from build123d import *

# Parameters (mm, degrees)
F0_W     = 76.2
F0_H     = 120.65
F0_R     = 2.5527
F1_DEPTH = 6.35
F2_R     = 9.525
F3_DEPTH = 6.35
F2_W     = 55.88
F2_H     = 43.18
F4_DEPTH = 5
F5_R     = 5.08
F6_W     = 69.85
F6_H     = 69.85
F6_W_2   = 62.23
F6_H_2   = 59.69
F7_DEPTH = 1.08458
F9_DEPTH = 5


# Not quite as in the source:
# - a length typed as a fraction of an inch, garbled in the dataset ("3 / 203.2 mm" for 3/8 in), is restored


with BuildPart() as f1:
    # F0 (on Top) → F1 (new body)
    with BuildSketch(Plane.XY):
        Rectangle(F0_W, F0_H)
        with Locations((-29.8323, -52.0573)):
            Circle(F0_R, mode=Mode.SUBTRACT)
        with Locations((29.8323, -52.0573)):
            Circle(F0_R, mode=Mode.SUBTRACT)
        with Locations((-29.8323, 52.0573)):
            Circle(F0_R, mode=Mode.SUBTRACT)
        with Locations((29.8323, 52.0573)):
            Circle(F0_R, mode=Mode.SUBTRACT)
    extrude(amount=F1_DEPTH)

    # F2 (on face) → F3 (cut)
    with BuildSketch(Plane.XY.offset(6.35)):
        Circle(F2_R)
    extrude(amount=-F3_DEPTH, mode=Mode.SUBTRACT)

    # F2 (on face) → F4 (cut)
    with BuildSketch(Plane.XY.offset(6.35)):
        with Locations((0, -1.27)):
            Rectangle(F2_W, F2_H)
        Circle(F2_R, mode=Mode.SUBTRACT)
    extrude(amount=-F4_DEPTH, mode=Mode.SUBTRACT)

    # F5
    f5_edges = [f1.edges().sort_by_distance(p)[0] for p in [
        (38.1, -60.325, 3.175),
        (38.1, 60.325, 3.175),
        (-38.1, 60.325, 3.175),
        (-38.1, -60.325, 3.175),
    ]]
    fillet(f5_edges, radius=F5_R)

    # F6 (on face) → F7 (cut)
    with BuildSketch(Plane.XY.offset(6.35)):
        Rectangle(F6_W, F6_H)
        Rectangle(F6_W_2, F6_H_2, mode=Mode.SUBTRACT)
    extrude(amount=-F7_DEPTH, mode=Mode.SUBTRACT)

    # F8 (on face) → F9 (cut)
    with BuildSketch(Plane.XY.offset(6.35)):
        Polygon((-25.7090758532, 20.32), (-20.905200392, 20.32), (-20.905200392, 22.5038137287), (27.94, 22.5038137287), (27.94, 26.3926647604), (-25.7090758532, 26.3926647604), align=None)
    extrude(amount=-F9_DEPTH, mode=Mode.SUBTRACT)


solid = f1.part
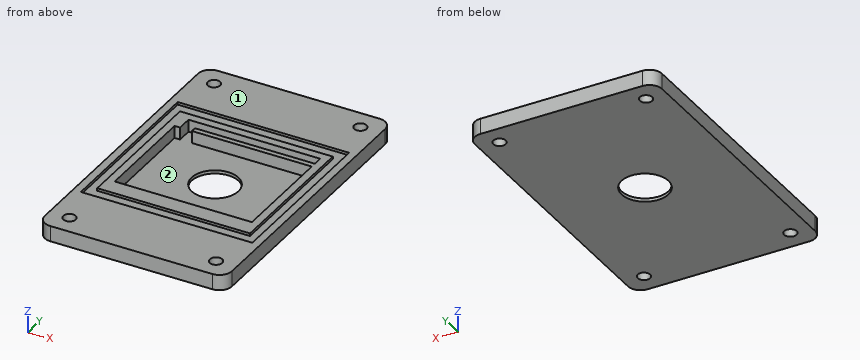
Design review of the part built by this model. Coordinates are the model's own, in mm. Face numbers are marked on the shaded views. Round coordinates to 2 decimals unless told otherwise and drop trailing zeros. Order: outer loops, then holes, each group sorted by start corner. A loop starts at its lowest first (then second) coordinate and runs counter-clockwise, first axis right, second up.
1) Consider section C-C (x = -11.5). State the section outline as (y, z) points (3 decimals).
The answers:
outline: (-60.325, 0) - (60.325, 0) - (60.325, 6.35) - (34.925, 6.35) - (34.925, 5.265) - (29.845, 5.265) - (29.845, 6.35) - (26.393, 6.35) - (26.393, 1.35) - (22.504, 1.35) - (22.504, 6.35) - (20.32, 6.35) - (20.32, 1.35) - (-22.86, 1.35) - (-22.86, 6.35) - (-29.845, 6.35) - (-29.845, 5.265) - (-34.925, 5.265) - (-34.925, 6.35) - (-60.325, 6.35) - close
2) Consider section A-A (y = 0). State the section outline as (x, z) points (3 decimals).
The answers:
outline: (-38.1, 0) - (-9.525, 0) - (-9.525, 1.35) - (-27.94, 1.35) - (-27.94, 6.35) - (-31.115, 6.35) - (-31.115, 5.265) - (-34.925, 5.265) - (-34.925, 6.35) - (-38.1, 6.35) - close; (9.525, 0) - (38.1, 0) - (38.1, 6.35) - (34.925, 6.35) - (34.925, 5.265) - (31.115, 5.265) - (31.115, 6.35) - (27.94, 6.35) - (27.94, 1.35) - (9.525, 1.35) - close
3) Consider section B-B (x = 0). State the section outline as (y, z) points (3 decimals).
The answers:
outline: (-60.325, 0) - (-9.525, 0) - (-9.525, 1.35) - (-22.86, 1.35) - (-22.86, 6.35) - (-29.845, 6.35) - (-29.845, 5.265) - (-34.925, 5.265) - (-34.925, 6.35) - (-60.325, 6.35) - close; (9.525, 0) - (60.325, 0) - (60.325, 6.35) - (34.925, 6.35) - (34.925, 5.265) - (29.845, 5.265) - (29.845, 6.35) - (26.393, 6.35) - (26.393, 1.35) - (22.504, 1.35) - (22.504, 6.35) - (20.32, 6.35) - (20.32, 1.35) - (9.525, 1.35) - close
4) For L1, parallel to Y at x = 0.5, z = 4.25 (3 decimals); L2, parallel to Y at x = -27, z = 4 (3 decimals); L3, parallel to X at y = 22, z = 1.5, list the stretches that pass through material, from the lowest coordinate up.
The answers:
L1: y = -60.325 to -22.86, 20.32 to 22.504, 26.393 to 60.325
L2: y = -60.325 to -22.86, 20.32 to 60.325
L3: x = -38.1 to -25.71, -20.91 to 38.1
5) Consider section D-D (z = 4.25). State the section outline as (x, y) points (3 decimals), plus the area to 3 significant figures.
The answers:
outline: (-38.1, -55.245) arc R5.08 ccw to (-33.02, -60.325) - (33.02, -60.325) arc R5.08 ccw to (38.1, -55.245) - (38.1, 55.245) arc R5.08 ccw to (33.02, 60.325) - (-33.02, 60.325) arc R5.08 ccw to (-38.1, 55.245) - close; hole circle Ø5.105 at (-29.832, -52.057); hole circle Ø5.105 at (-29.832, 52.057); hole (-27.94, -22.86) - (27.94, -22.86) - (27.94, 20.32) - (-20.905, 20.32) - (-20.905, 22.504) - (27.94, 22.504) - (27.94, 26.393) - (-25.709, 26.393) - (-25.709, 20.32) - (-27.94, 20.32) - close; hole circle Ø5.105 at (29.832, -52.057); hole circle Ø5.105 at (29.832, 52.057)
area: 6,460 mm2
6) Clearance check with a flat-ended pin moving along its axis: pin 1 Ø1.5 at (x, y) = (-6.5, 6.5) entering from +Z. State where the tip first meets the part, or that it passes through.
The answers:
pin 1: stops at z = 1.35
7) Draft analysis for pull direction X (two halves, no side actions). For the marked faces 1 and 2, state which applies: released by +X, released by -X, zero draft, split by the parting line, or undercut.
The answers:
face 1: zero draft
face 2: undercut
